from build123d import *

# Parameters (mm, degrees)
SKETCH1_W               = 23
SKETCH1_H               = 15
BOSS_EXTRUDE1_DEPTH     = 20
SKETCH2_W               = 11
SKETCH2_H               = 15
CUT_EXTRUDE1_DEPTH      = 15
CUT_EXTRUDE2_DEPTH      = 34.970575503
CUT_EXTRUDE2_DEPTH_BACK = 34.970575503
SKETCH3_R               = 1.7
CHAMFER1_SIZE           = 2.5
CHAMFER1_SIZE_2         = 14.178204549
SKETCH4_R               = 2.2
CUT_EXTRUDE3_DEPTH      = 10
CUT_EXTRUDE4_DEPTH      = 2
SKETCH6_R               = 3.25
CUT_EXTRUDE5_DEPTH      = 2.5
CUT_EXTRUDE6_DEPTH      = 3.8
CHAMFER3_SIZE           = 1
SKETCH9_R               = 1.85
SKETCH9_R_2             = 1.6
BOSS_EXTRUDE2_DEPTH     = 1
BOSS_EXTRUDE3_START     = 1
SKETCH8_R               = 1.85
SKETCH8_R_2             = 1.600864578
BOSS_EXTRUDE3_DEPTH     = 1
CHAMFER4_SIZE           = 1
BOSS_EXTRUDE4_START     = -17
SKETCH10_W              = 20
SKETCH10_H              = 1
BOSS_EXTRUDE4_DEPTH     = 11


# Some blends are built 0.0001 mm under size
with BuildPart() as part:
    # Sketch1 → Boss-Extrude1 (new body)
    with BuildSketch(Plane(origin=(0, 0, 0), x_dir=(0, 0, -1), z_dir=(1, 0, 0))):
        with Locations((11.5, 7.5)):
            Rectangle(SKETCH1_W, SKETCH1_H)
    extrude(amount=BOSS_EXTRUDE1_DEPTH)

    # Sketch2 → Cut-Extrude1 (cut)
    with BuildSketch(Plane(origin=(20, 0, 0), x_dir=(0, 0, -1), z_dir=(1, 0, 0))):
        with Locations((11.5, 7.5)):
            Rectangle(SKETCH2_W, SKETCH2_H)
    extrude(amount=-CUT_EXTRUDE1_DEPTH, mode=Mode.SUBTRACT)

    # Sketch3 → Cut-Extrude2 (cut, two sides: drawn at the far end of the back side and taken through both)
    with BuildSketch(Plane(origin=(0, 0, -23), x_dir=(-1, 0, 0), z_dir=(0, 0, -1)).offset(-CUT_EXTRUDE2_DEPTH_BACK)):
        with Locations(Location((-16, 9.5, 0), (0, 0, 90))):
            Circle(SKETCH3_R)
    extrude(amount=CUT_EXTRUDE2_DEPTH + CUT_EXTRUDE2_DEPTH_BACK, mode=Mode.SUBTRACT)

    # Chamfer1
    # the kernel refuses this chamfer: 14.178204549, 2.5 mm, written as the material it takes off along each edge
    with BuildSketch(Plane(origin=(0, 15, -59.842614584), x_dir=(-0.21013876076743537, -0.9776715712462578, 0), z_dir=(0, 0, 1))) as chamfer1_piece_1:
        Polygon((CHAMFER1_SIZE * 0.977671571246, CHAMFER1_SIZE * 0.210138760767), (-CHAMFER1_SIZE_2 * 0.210138760768, CHAMFER1_SIZE_2 * 0.977671571249), (0, 0), align=None)
    extrude(amount=96.685229169, mode=Mode.SUBTRACT)

    # Sketch4 → Cut-Extrude3 (cut)
    with BuildSketch(Plane.ZY):
        with Locations((-11.5, 6.25)):
            Circle(SKETCH4_R)
    extrude(amount=-CUT_EXTRUDE3_DEPTH, mode=Mode.SUBTRACT)

    # Sketch5 → Cut-Extrude4 (cut)
    with BuildSketch(Plane(origin=(5, 0, 0), x_dir=(0, 0, -1), z_dir=(1, 0, 0))):
        Polygon((7.9, 8.328460969), (7.9, 4.171539031), (11.5, 2.093078062), (15.1, 4.171539031), (15.1, 8.328460969), (11.5, 10.406921938), align=None)
    extrude(amount=-CUT_EXTRUDE4_DEPTH, mode=Mode.SUBTRACT)

    # Sketch6 → Cut-Extrude5 (cut)
    with BuildSketch(Plane(origin=(0, 0, -23), x_dir=(-1, 0, 0), z_dir=(0, 0, -1))):
        with Locations((-16, 9.5)):
            Circle(SKETCH6_R)
    extrude(amount=-CUT_EXTRUDE5_DEPTH, mode=Mode.SUBTRACT)

    # Sketch7 → Cut-Extrude6 (cut)
    with BuildSketch(Plane.XY):
        Polygon((13.1, 11.174315781), (13.1, 7.825684219), (16, 6.151368439), (18.9, 7.825684219), (18.9, 11.174315781), (16, 12.848631561), align=None)
    extrude(amount=-CUT_EXTRUDE6_DEPTH, mode=Mode.SUBTRACT)

    # Chamfer3
    chamfer3_edges = [part.edges().sort_by_distance(p)[0] for p in [
        (5, 6.690817452, -17),
        (5, 6.690817452, -6),
    ]]
    chamfer(chamfer3_edges, length=CHAMFER3_SIZE)

    # Sketch9 → Boss-Extrude2 (add)
    with BuildSketch(Plane(origin=(0, 0, -6), x_dir=(-1, 0, 0), z_dir=(0, 0, -1))):
        with Locations(Location((-16, 9.5, 0), (0, 0, 270))):
            Circle(SKETCH9_R)
        with Locations(Location((-16, 9.5, 0), (0, 0, 90))):
            Circle(SKETCH9_R_2, mode=Mode.SUBTRACT)
    extrude(amount=BOSS_EXTRUDE2_DEPTH)

    # Sketch8 → Boss-Extrude3 (add)
    with BuildSketch(Plane.XY.offset(-17).offset(BOSS_EXTRUDE3_START)):
        with Locations(Location((16, 9.5, 0), (0, 0, 270))):
            Circle(SKETCH8_R)
        with Locations((16, 9.5)):
            Circle(SKETCH8_R_2, mode=Mode.SUBTRACT)
    extrude(amount=-BOSS_EXTRUDE3_DEPTH)

    # Chamfer4
    chamfer4_edges = [part.edges().sort_by_distance(p)[0] for p in [
        (16, 11.35, -6),
        (16, 11.35, -17),
    ]]
    chamfer(chamfer4_edges, length=CHAMFER4_SIZE - 0.0001)  # a hair under: the kernel refuses the full size

    # Sketch10 → Boss-Extrude4 (add)
    with BuildSketch(Plane(origin=(0, 0, -23), x_dir=(-1, 0, 0), z_dir=(0, 0, -1)).offset(BOSS_EXTRUDE4_START)):
        with Locations((-10, 0.5)):
            Rectangle(SKETCH10_W, SKETCH10_H)
    extrude(amount=BOSS_EXTRUDE4_DEPTH)


solid = part.part
Verification items for the finished model (mm, model axes). A direction names the side the tool comes from. Round coordinates to 2 decimals unless told otherwise and drop trailing zeros. Loops run counter-clockwise (first coordinate to the right, second up) from the corner with the lowest first, then second, coordinate; pieces in that order, holes last. Notation, with made-up numbers: (-17, 6) - (-1, 6) arc R6 ccw to (-1, 12) - close; hole circle Ø2 at (6.5, 18). An arc over 180 degrees is marked (long way). Use one line per item in the form item = value.
1. Section check B-B on x = 6.75. Record the cut outline in (y, z), and give its area (3 significant figures).
A:
outline = (0, -23) - (13.69, -23) - (13.69, -17) - (1, -17) - (1, -6) - (13.69, -6) - (13.69, 0) - (0, 0) - close
area = 175 mm²
2. Gauge pin test, flat ends, axial feed: pin 1 Ø7 at (y, z) = (5, -11) entering from +X; pin 2 Ø4 at (x, y) = (16, 9.5) entering from +Z; pin 3 Ø1.9 at (x, y) = (16, 9.5) entering from -Z; pin 4 Ø3.5 at (x, y) = (17, 9.5) entering from -Z. Record the tip position at first contact, or that the pin passes through.
A:
pin_1 = 5
pin_2 = -3.8
pin_3 = through
pin_4 = -20.5
3. Access from +Z, -Z, +X, -X, +Y, -Y to the whole of each face (thin tool, end or side, straight path). Record for faces 1 (the flat face through (4.014, 9.382, -9.725)), 2 (the flat face through (13.1, 10, -2)), 3 (the flat face through (5.5, 7.2, -16.5)).
A:
face_1 = +X
face_2 = +Z
face_3 = +Y
4. Section check A-A on y = 5.75. Record the cut outline in (x, z).
A:
outline = (0, -23) - (20, -23) - (20, -17) - (6, -17) - (5, -16) - (5, -15.1) - (3, -15.1) - (3, -13.64) - (0, -13.64) - close; (0, -9.36) - (3, -9.36) - (3, -7.9) - (5, -7.9) - (5, -7) - (6, -6) - (20, -6) - (20, 0) - (0, 0) - close
5. Section check C-C on z = -15.5. Record the cut outline in (x, y).
A:
outline = (0, 0) - (20, 0) - (20, 1) - (5, 1) - (5, 13.38) - (0, 12.5) - close
6. Draft check along Y on faces 4 (the flat face through (10, 0, -11)), 5 (the flat face through (20, 0.7, -11.3)), 6 (the flat face through (14.57, 12.023, -1.873)). Enter one of: pulls with the +Y half, pulls with the -Y half, needs draft (parallel to the pull), parting line crosses it, or undercut.
A:
face_4 = pulls with the -Y half
face_5 = needs draft
face_6 = undercut
7. Section check D-D on x = 4.25. Record the cut outline in (y, z), and give its area (3 significant figures).
A:
outline = (0, -23) - (13.25, -23) - (13.25, 0) - (0, 0) - close; hole (2.09, -11.5) - (4.17, -15.1) - (8.33, -15.1) - (10.41, -11.5) - (8.33, -7.9) - (4.17, -7.9) - close
area = 260 mm²
8. Scan lines: probe 1 along Z at (x, y) = (8, 9.25); probe 2 along X at (y, z) = (9, -3.5); probe 3 along X at (y, z) = (9.5, -6.55). Record each from-to range of solid material in increasing order.
A:
probe_1 = -23 to -17, -6 to 0
probe_2 = 0 to 13.1, 18.9 to 20
probe_3 = 0 to 5.45, 13.7 to 14.4, 17.6 to 18.3
